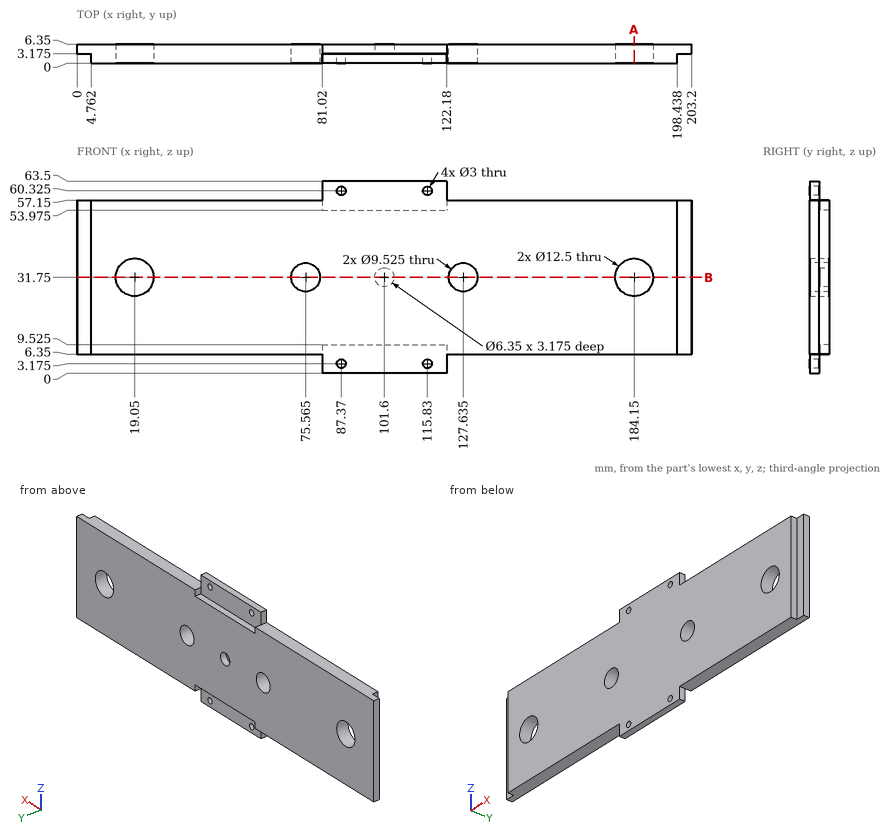
Print and shaded views of the part. All mm, measured from the part's lowest x, y and z. Give positions to 0.01 mm unless a question says otherwise; leave off trailing zeros. Loops run counter-clockwise (first coordinate to the right, second up) from the corner with the lowest first, then second, coordinate; pieces in that order, holes last. Notation, with made-up numbers: (-7, -40) - (50, -40) arc R16 cw to (50, -14) - close; hole circle Ø11 at (20.25, 18). An arc over 180 degrees is marked (long way). One line per item, written item: value. Start each with the question number.
1. Probe L1, parallel to Z at x = 115.83, y = 1.25 (1 decimal); L2, parallel to X at y = 3.75, z = 31.75 (1 decimal); L3, parallel to X at y = 3.75, z = 31 (1 decimal). List the from-to ranges inside material, lowest first. Write a range as from..to.
2. Pin check, flat tips, straight feed: pin 1 (1.9 mm diameter, centred on x = 169, y = 4, fed in from -Z); pin 2 (4 mm diameter, centred on x = 1.5, z = 24, fed in from -Y) (1 decimal); pin 3 (2.5 mm diameter, centred on x = 100.5, y = 5.5, fed in from +Z) (1 decimal). Stop position of each tip, or through.
3. Slice it at A-A (x = 184.15). List the corners of the cut face in (y, z).
4. Slice it at B-B (z = 31.75). Give the number of separate pieces and of enclosed holes in the cut face.
Solution:
1. L1: z = 0..1.7, 4.7..58.8, 61.8..63.5
1. L2: x = 0..12.8, 25.3..70.8, 80.3..98.4, 104.8..122.9, 132.4..177.9, 190.4..203.2
1. L3: x = 0..12.8, 25.3..70.9, 80.3..98.5, 104.7..122.9, 132.3..177.9, 190.4..203.2
2. pin 1: stops at z = 6.35
2. pin 2: stops at y = 3.2
2. pin 3: stops at z = 54
3. outline: (0, 6.35) - (6.35, 6.35) - (6.35, 25.5) - (0, 25.5) - close; (0, 38) - (6.35, 38) - (6.35, 57.15) - (0, 57.15) - close
4. separate pieces: 5
4. enclosed holes: 0
